```python
from build123d import *

# Parameters (mm, degrees)
CHAMFER1_SIZE = 0.381
FILLET1_R     = 0.508


with BuildPart() as part:
    # Sketch1 → Revolve1 (revolve)
    with BuildSketch(Plane.XY, mode=Mode.PRIVATE) as revolve1_sk:
        Polygon((2.413, 0.762), (8.763, 0.762), (9.525, 0), (14.2875, 0), (14.2875, 12.7), (11.1125, 12.7), (2.413, 4.0005), align=None)
    revolve(revolve1_sk.sketch.rotate(Axis((0, 0, 0), (0, 1, 0)), 90), axis=Axis((0, 0, 0), (0, 1, 0)))  # turned: the seam where the file's is

    # Chamfer1
    chamfer1_edges = [part.edges().sort_by_distance(p)[0] for p in [
        (0, 0.762, 2.413),
    ]]
    chamfer(chamfer1_edges, length=CHAMFER1_SIZE)

    # Fillet1
    fillet1_edges = [part.edges().sort_by_distance(p)[0] for p in [
        (0, 0, 14.2875),
        (0, 12.7, 14.2875),
        (0, 12.7, 11.1125),
    ]]
    fillet(fillet1_edges, radius=FILLET1_R)


solid = part.part
```
Here's how the part is built. I have some questions about the finished solid (model axes, mm). Coordinates: 2 decimals unless noted, no trailing zeros. Order: outer loops, then holes, each group sorted by start corner. A loop starts at its lowest first (then second) coordinate and runs counter-clockwise, first axis right, second up. Notation, with made-up numbers: (-31, 7.25) - (0, 7.25) arc R20 cw to (0, 19.25) - close; hole circle Ø11 at (81.5, 69). An arc over 180 degrees is marked (long way). One line per question, with ' | ' between items. Start each with the question number.
1. If we section it at D-D (y = 6): Write out the boundary of the cut face in (x, z) (1 decimal).
2. If we mould it in two halves opening along X, with no side actions, what happens to faces 1 (the flat face through (-9.4, 0, 2.9)), 2 (the flat face through (-2.1, 0.762, -2.1)), 3 (the cylindrical face through (-0.628, 6.432, 14.274))? For each: released by +X, released by -X, zero draft, split by the parting line, or undercut.
3. If we section it at C-C (y = 8.25): Write out the boundary of the cut face in (x, z) (1 decimal).
4. I'm going to push flat-ended pins straight in: pin 1 Ø4 at (x, y) = (7.5, 10.5) entering from +Z; pin 2 Ø1 at (x, z) = (8.5, -9) entering from -Y; pin 3 Ø2 at (x, y) = (-3, 8.5) entering from +Z; pin 4 Ø7.5 at (x, z) = (0, 0) entering from +Y. Where does each tip first touch, or does it pass through?
5. Please list where these lines run through material, in increasing order: line 1 along X through (y, z) = (3.3, 0); line 2 along Z through (x, y) = (-3.5, 6.75); line 3 along Z through (x, y) = (-3.25, 8.5). Write a range as [from, to].
Model answer:
1) outline: circle Ø28.6 at (0, 0); hole circle Ø8.8 at (0, 0)
2) face 1: zero draft | face 2: undercut | face 3: split by the parting line
3) outline: circle Ø28.6 at (0, 0); hole circle Ø13.3 at (0, 0)
4) pin 1: stops at z = 13.19 | pin 2: stops at y = 0 | pin 3: stops at z = 14.15 | pin 4: stops at y = 5.34
5) line 1: x = [-14.29, -2.41], [2.41, 14.29] | line 2: z = [-13.85, -3.79], [3.79, 13.85] | line 3: z = [-13.91, -6.1], [6.1, 13.91]
